Part print with two shaded views. Sizes in mm from the minimum x, y, z corner. Give positions to 0.01 mm unless a question says otherwise; leave off trailing zeros. Write each loop counter-clockwise with the first axis right and the second up, starting at its lowest first coordinate (ties: lowest second). Pieces come first, ordered by that corner, then holes.
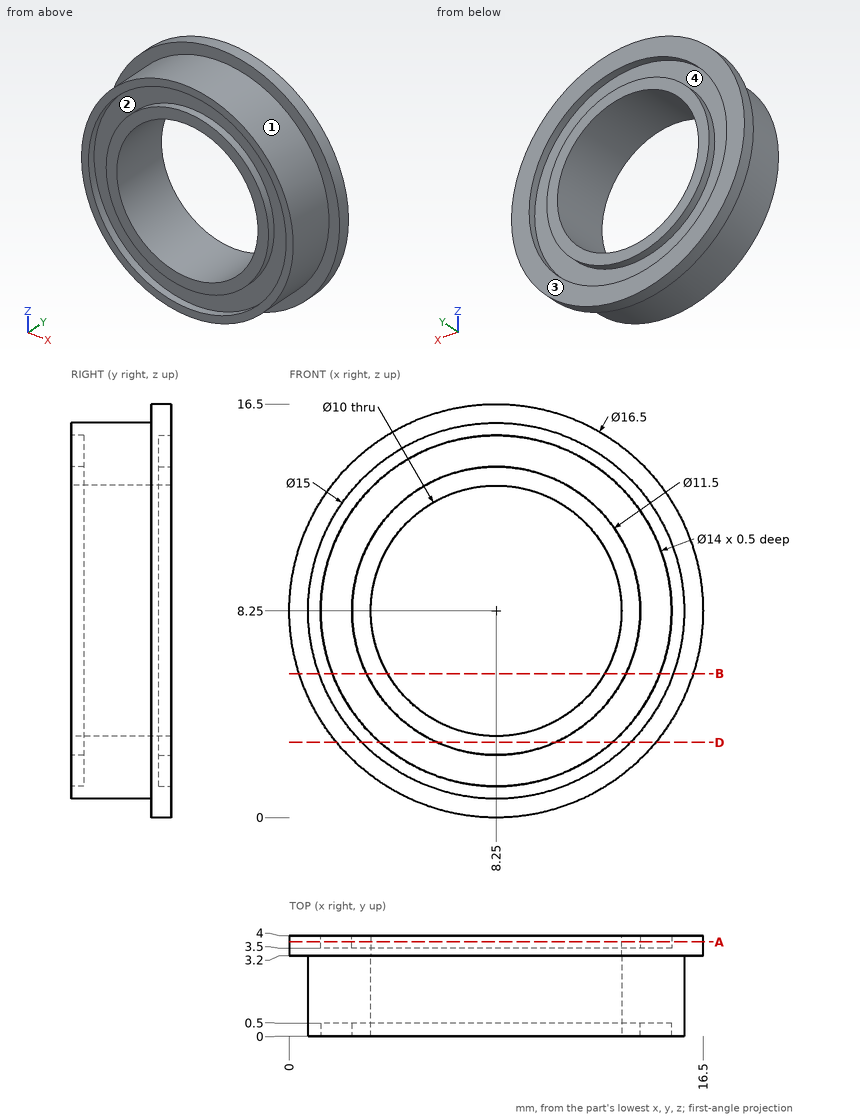
1) Two-plate mould, pull along X, no slides. Class the marked faces 1, 2, 3 and 4: +X half, -X half, draft (parallel to the pull), parting line (faces both ways), or undercut.
Answers follow:
face 1: parting line
face 2: undercut
face 3: draft
face 4: undercut
2) Wall check: L1, parallel to Z at x = 8.25, y = 3.7; L2, parallel to Z at x = 8.25, y = 0.4; L3, parallel to Z at x = 8.25, y = 2.15. Give the ranges that are in metal, low to high.
Answers follow:
L1: z = 0 to 1.25, 2.5 to 3.25, 13.25 to 14, 15.25 to 16.5
L2: z = 0.75 to 1.25, 2.5 to 3.25, 13.25 to 14, 15.25 to 15.75
L3: z = 0.75 to 3.25, 13.25 to 15.75
3) Pin check, flat tip, straight feed: pin 1 Ø5 at (x, z) = (9.5, 8.5) entering from -Y. Stop position of the tip, or through.
Answers follow:
pin 1: passes through
4) Saw through at A-A, the plane y = 3.75. Write the cut outline in (x, z), then the cut area to 3 significant figures.
Answers follow:
outline: circle Ø16.5 at (8.25, 8.25); circle Ø11.5 at (8.25, 8.25); hole circle Ø14 at (8.25, 8.25); hole circle Ø10 at (8.25, 8.25)
area: 85.2 mm2
5) Saw through at D-D, the plane z = 3. Write the cut outline in (x, y).
Answers follow:
outline: (1.89, 3.2) - (2.89, 3.2) - (2.89, 0) - (3.62, 0) - (3.62, 0.5) - (5.9, 0.5) - (5.9, 0) - (10.6, 0) - (10.6, 0.5) - (12.88, 0.5) - (12.88, 0) - (13.61, 0) - (13.61, 3.2) - (14.61, 3.2) - (14.61, 4) - (12.88, 4) - (12.88, 3.5) - (10.6, 3.5) - (10.6, 4) - (5.9, 4) - (5.9, 3.5) - (3.62, 3.5) - (3.62, 4) - (1.89, 4) - close
6) Saw through at B-B, the plane z = 5.75. Write the cut outline in (x, y).
Answers follow:
outline: (0.39, 3.2) - (1.18, 3.2) - (1.18, 0) - (1.71, 0) - (1.71, 0.5) - (3.07, 0.5) - (3.07, 0) - (3.92, 0) - (3.92, 4) - (3.07, 4) - (3.07, 3.5) - (1.71, 3.5) - (1.71, 4) - (0.39, 4) - close; (12.58, 0) - (13.43, 0) - (13.43, 0.5) - (14.79, 0.5) - (14.79, 0) - (15.32, 0) - (15.32, 3.2) - (16.11, 3.2) - (16.11, 4) - (14.79, 4) - (14.79, 3.5) - (13.43, 3.5) - (13.43, 4) - (12.58, 4) - close
